```python
from build123d import *

# Parameters (mm, degrees)
BOSS_EXTRUDE1_DEPTH = 30
SHELL13_T           = -3
SKETCH3_R           = 3
CUT_EXTRUDE2_DEPTH  = 3
SKETCH4_W           = 10
SKETCH4_H           = 1
SKETCH4_W_2         = 1
SKETCH4_H_2         = 10
SKETCH4_W_3         = 7
CUT_EXTRUDE3_DEPTH  = 5


with BuildPart() as part:
    # Sketch1 → Boss-Extrude1 (new body)
    with BuildSketch(Plane.XY):
        with BuildLine():
            Line((15, -15), (15, 15))
            Line((15, 15), (-15, 15))
            Line((-15, 15), (-15, -15))
            ThreePointArc((-15, -15), (0, -19.004680178), (15, -15))
        make_face()
    extrude(amount=BOSS_EXTRUDE1_DEPTH)

    # Shell13
    shell13_openings = [part.faces().sort_by_distance(p)[0] for p in [
        (0, -1.375060702, 0),
    ]]
    offset(amount=SHELL13_T, openings=shell13_openings, kind=Kind.INTERSECTION)

    # Sketch3 → Cut-Extrude2 (cut)
    with BuildSketch(Plane(origin=(0, 0, 27), x_dir=(-1, 0, 0), z_dir=(0, 0, -1))):
        with Locations((0.010259738, 0.007572697)):
            Circle(SKETCH3_R)
    extrude(amount=-CUT_EXTRUDE2_DEPTH, mode=Mode.SUBTRACT)

    # Sketch4 → Cut-Extrude3 (cut)
    with BuildSketch(Plane(origin=(0, 0, 0), x_dir=(-1, 0, 0), z_dir=(0, 0, -1))):
        with Locations((0, 13.5)):
            Rectangle(SKETCH4_W, SKETCH4_H)
        with Locations((-13.5, 0)):
            Rectangle(SKETCH4_W_2, SKETCH4_H_2)
        with Locations((0, -17.5)):
            Rectangle(SKETCH4_W_3, SKETCH4_H)
        with Locations((13.5, 0)):
            Rectangle(SKETCH4_W_2, SKETCH4_H_2)
    extrude(amount=-CUT_EXTRUDE3_DEPTH, mode=Mode.SUBTRACT)


solid = part.part
```
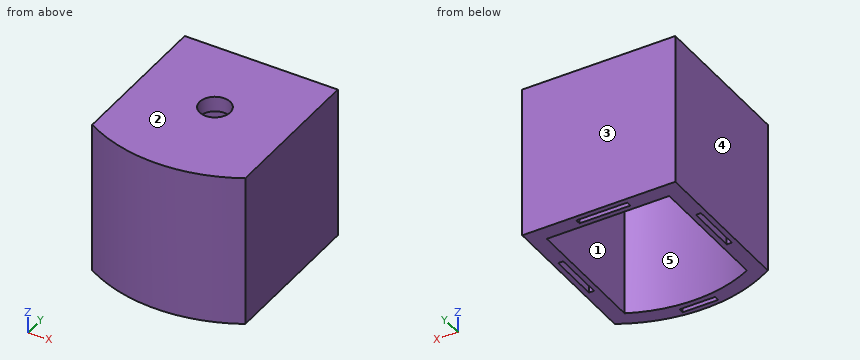
CAD build for the part. Positions are in the model's coordinates, mm. Face numbers are marked on the shaded views. A direction names the side the tool comes from. Round coordinates to 2 decimals unless told otherwise and drop trailing zeros. Write each loop counter-clockwise with the first axis right and the second up, starting at its lowest first coordinate (ties: lowest second). Pieces come first, ordered by that corner, then holes. Notation, with made-up numbers: M 55.25,-5.75 L 101.25,-5.75 A15 cw 101.25,18.25 Z; hole C -17,0 d5. An arc over 180 degrees is marked long. One line per question, with ' | ' between items.
1. Which spindle directions (+Z, -Z, +X, -X, +Y, -Y) get a long thin tool onto all of the face, cutting with end or side? Do the marked faces 1 and 2. Say none if no direction does.
Working result:
face 1: -Z | face 2: +Z, +X, -X, +Y, -Y
2. Cut at D-D on y = 1.5. Write the cut outline in (x, z), and give its area (3 significant figures).
Working result:
outline: M -15,0 L -14,0 L -14,5 L -13,5 L -13,0 L -12,0 L -12,27 L -2.61,27 L -2.61,30 L -15,30 Z; M 2.59,27 L 12,27 L 12,0 L 13,0 L 13,5 L 14,5 L 14,0 L 15,0 L 15,30 L 2.59,30 Z | area: 226 mm2
3. Probe L1, parallel to X at y = 3.5, z = 4.25; L2, parallel to Y at x = 4.5, z = 2.5; L3, parallel to X at y = 7, z = 21. List the from-to ranges inside material, lowest first. Write a range as from..to.
Working result:
L1: -15..-14, -13..-12, 12..13, 14..15 | L2: -18.67..-15.63, 12..13, 14..15 | L3: -15..-12, 12..15
4. Cut at C-C on z = 14. Write the cut outline in (x, y), and give its area (3 significant figures).
Working result:
outline: M -15,-15 A30.09 ccw 15,-15 L 15,15 L -15,15 Z; hole M -12,-13.2 A27.09 ccw 12,-13.2 L 12,12 L -12,12 Z | area: 331 mm2
5. Mould opens along Y. For the marked faces 3, 4 and 5 say: pulls with the +Y half, pulls with the -Y half, needs draft (parallel to the pull), parting line crosses it, or undercut.
Working result:
face 3: pulls with the +Y half | face 4: needs draft | face 5: undercut
6. Cut at B-B on y = -4.5. Write the cut outline in (x, z), and give its area (3 significant figures).
Working result:
outline: M -15,0 L -14,0 L -14,5 L -13,5 L -13,0 L -12,0 L -12,27 L 12,27 L 12,0 L 13,0 L 13,5 L 14,5 L 14,0 L 15,0 L 15,30 L -15,30 Z | area: 242 mm2
7. Pin check, flat tips, straight feed: pin 1 Ø5 at (x, z) = (0, 14.5) entering from -Y; pin 2 Ø0.5 at (x, y) = (-13.5, -0.5) entering from -Z; pin 3 Ø12 at (x, y) = (-4.5, 1.5) entering from -Z. Stop position of each tip, or through.
Working result:
pin 1: y = -19 | pin 2: z = 5 | pin 3: z = 27
8. Cut at A-A on z = 3.5. Write the cut outline in (x, y).
Working result:
outline: M -15,-15 A30.09 ccw 15,-15 L 15,15 L -15,15 Z; hole M -14,-5 L -13,-5 L -13,5 L -14,5 Z; hole M -12,-13.2 A27.09 ccw 12,-13.2 L 12,12 L -12,12 Z; hole M -5,13 L 5,13 L 5,14 L -5,14 Z; hole M -3.5,-18 L 3.5,-18 L 3.5,-17 L -3.5,-17 Z; hole M 13,-5 L 14,-5 L 14,5 L 13,5 Z
